Autodesk Inventor part; units mm, degrees
ref_plane "Плоскость сечения" through (-16.6855, 62.9464, 0) normal (-0.21, -0.9777, 0) x (0, 0, 1)
ref_plane "РабПлоскость2" through (14.9336, 56.1551, 0) normal (-1, 0, 0) x (0, 0, 1)
ref_plane "РабПлоскость3" through (170, -200, 0) normal (-0.5674, 0.8234, 0) x (0, 0, 1)
sketch "Эскизная траектория" plane through (0, 0, 0) normal (0, 0, 1) x (1, 0, 0)
  arc A0 (41.531, 74.5528) -> (-16.6855, 62.9464) centre (14.9336, 56.1551) ccw
  arc A1 (144.3794, -243.555) -> (211.5583, -171.2536) centre (170, -200) ccw
  arc A2 (-49.4049, -89.3885) -> (-25.6206, -143.555) centre (0, -100) ccw
  line L0 (-49.4049, -89.3885) -> (-16.6855, 62.9464)
  line L1 (41.531, 74.5528) -> (211.5583, -171.2536)
  line L2 (144.3794, -243.555) -> (-25.6206, -143.555)
ref_plane "Плоскость сечения" through (-16.6855, 62.9464, 0) normal (-0.21, -0.9777, 0) x (0, 0, 1)
ref_plane "РабПлоскость2" through (14.9336, 56.1551, 0) normal (-1, 0, 0) x (0, 0, 1)
ref_plane "РабПлоскость3" through (170, -200, 0) normal (-0.5674, 0.8234, 0) x (0, 0, 1)
ref_plane "РабПлоскость4" through (0, -100, 0) normal (0.7593, -0.6507, 0) x (0, 0, 1)
sketch "Сечение" plane through (-16.6855, 62.9464, 0) normal (-0.21, -0.9777, 0) x (0, 0, 1)
  line L0 (-9.525, 1.3462) -> (9.525, 1.3462)
  line L1 (9.525, 1.3462) -> (9.525, -0.6858)
  line L2 (9.525, -0.6858) -> (-9.525, -0.6858)
  line L3 (-9.525, -0.6858) -> (-9.525, 1.3462)
  line L4 (-9.525, 0) -> (9.525, 0) construction
  point P0 (0, 0)
  point P1 (0, 0)
  dimension "d0" = 19.05
  dimension "d4" = 0.6858
  dimension "d5" = 1.3462
sweep "Ремень" add profiles "Сечение" path "Эскизная траектория"
equation "\"d0\" = da_B"
equation "\"d4\" = da_a"
equation "\"d5\" = da_a2"
equation "\"da_B\" = 19.05"
equation "\"da_pb\" = 12.7"
equation "\"da_L\" = 927.12858"
equation "\"da_a\" = 0.6858"
equation "\"da_S\" = 6.1214"
equation "\"da_Beta\" = 20deg"
equation "\"da_Ht\" = 2.286"
equation "\"da_H\" = 4.318"
equation "\"da_a2\" = 1.3462"
properties part number "Зубчатый ремень" material "Rubber"
Read the model definition and answer for the solid it produces. Units are mm, in the model's axes. A direction names the side the tool comes from. Round coordinates to 2 decimals unless told otherwise and drop trailing zeros. Loops run counter-clockwise (first coordinate to the right, second up) from the corner with the lowest first, then second, coordinate; pieces in that order, holes last. Notation, with made-up numbers: (18, -34.75) - (39, -34.75) arc R14 cw to (39, -7.75) - close; hole circle Ø11 at (-25.75, 51.25). An arc over 180 degrees is marked (long way). One line per question, with ' | ' between items. Start each with the question number.
Q1. Section C-C on y = -128 is taken. Give the vertices of the cut face in (x, z) (3 decimals), plus the area to 3 significant figures.
Q2. Section B-B on x = 66.5 is taken. Give the vertices of the cut face in (y, z) (3 decimals), plus the area to 3 significant figures.
Q3. Flat-ended cylindrical pins translate along their axes: pin 1 (4 mm diameter, centred on y = -44.5, z = 6.5, fed in from -X); pin 2 (3 mm diameter, centred on y = -168.5, z = -3.5, fed in from +X); pin 3 (1 mm diameter, centred on x = 69.5, z = 3.5, fed in from -Y). Find the tip coordinate at first contact, or state that the pin passes through.
Q4. For a pull along X with two mould halves and no side action, classify faces 3 (the flat face through (-34.59, -14, 0.13)), 4 (the flat face through (-32.604, -14.431, -0.133)), 5 (the cylindrical face through (208.667, -234.586, -0.133)) as +X half, -X half, draft (parallel to the pull), parting line (faces both ways), or undercut.
Q5. Find the intervals of material crossed by L1, parallel to X at y = -161.5, z = -5.75; L2, parallel to X at y = 31, z = 8; L3, parallel to Y at x = 181, z = 1.5, in increasing order.
Q6. Section A-A on z = 2.75 is taken. Give the vertices of the cut face in (x, y) (3 decimals), plus the area to 3 significant figures.
Q7. For faces 1 (the flat face through (60.917, -193.664, -0.133)), 2 (the flat face through (126.46, -45.86, 0.13)), determine the directions among +Z, -Z, +X, -X, +Y, -Y from which every point of the face is accessible in a straight line to the end or side of a thin tool.
Established:
1) outline: (-43.673, -9.525) - (-41.238, -9.525) - (-41.238, 9.525) - (-43.673, 9.525) - close; (180.805, -9.525) - (183.276, -9.525) - (183.276, 9.525) - (180.805, 9.525) - close | area: 93.4 mm²
2) outline: (-199.305, -9.525) - (-196.948, -9.525) - (-196.948, 9.525) - (-199.305, 9.525) - close; (37.25, -9.525) - (40.822, -9.525) - (40.822, 9.525) - (37.25, 9.525) - close | area: 113 mm²
3) pin 1: x = -41.57 | pin 2: x = 212.33 | pin 3: y = -201.36
4) face 3: -X half | face 4: undercut | face 5: parting line
5) L1: 2.23 to 6.24, 203.98 to 206.45 | L2: -24.92 to -22.85, 70.82 to 73.29 | L3: -250.7 to -248.62, -128.28 to -124.71
6) outline: (-50.721, -89.106) arc R51.878 ccw to (-26.303, -144.715) - (143.697, -244.715) arc R51.878 ccw to (212.665, -170.488) - (42.638, 75.319) arc R33.686 ccw to (-18.002, 63.229) - close; hole (-48.734, -89.533) arc R49.846 ccw to (-25.273, -142.964) - (144.727, -242.964) arc R49.846 ccw to (210.994, -171.644) - (40.967, 74.163) arc R31.654 ccw to (-16.015, 62.802) - close | area: 1,890 mm²
7) face 1: +Z, -Z | face 2: +Z, -Z, +X, +Y
